Can you work these out from the drawing? Everything is in mm from the part's minimum corner. Coordinates: 2 decimals unless noted, no trailing zeros. Order: outer loops, then holes, each group sorted by start corner. A loop starts at its lowest first (then second) coordinate and runs counter-clockwise, first axis right, second up. Notation, with made-up numbers: M 11,11 L 25,11 A7 ccw 25,19 Z; hole C 85.5,20 d9. An arc over 180 degrees is marked long. Answer as CSV lines item,"result". Start each with the question number.
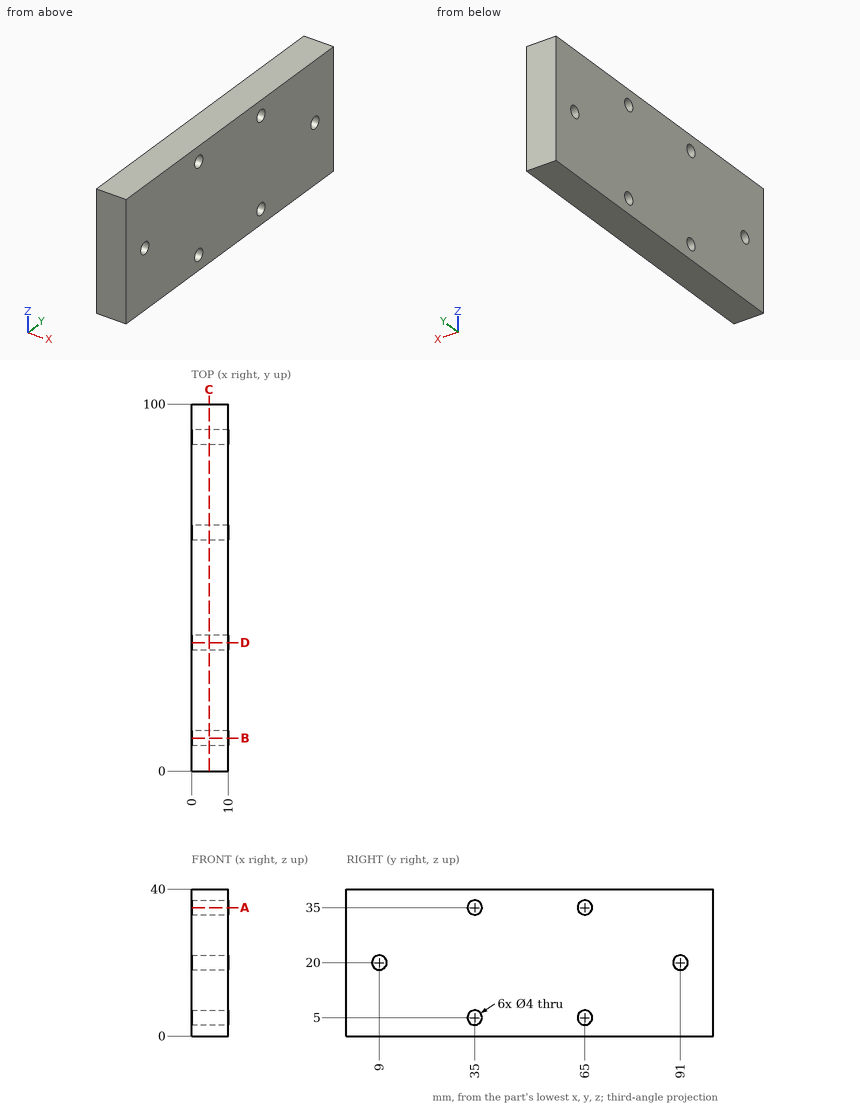
1) Suppose I cut it at B-B on y = 9. Please give me the cut outline in (x, z), plus the area to 3 significant figures.
2) Suppose I cut it at A-A on z = 35. Please give me the cut outline in (x, y).
3) Suppose I cut it at D-D on y = 35. Please give me the cut outline in (x, z), plus the area to 3 significant figures.
4) I need wall thicknesses on line 1 (Z direction, x = 4.5, y = 65); line 2 (Z direction, x = 7.25, y = 9); line 3 (Y direction, x = 1.5, z = 19.5). Which ranges of each line are inside material? Lowest first, please. Write a range as [from, to].
5) Suppose I cut it at C-C on x = 4.75. Please give me the cut outline in (y, z).
6) Will this pin go through, and if not, where does the flat tip stop? pin 1 Ø2.5 at (y, z) = (35, 5) entering from -X.
Output:
1,outline,"M 0,0 L 10,0 L 10,18 L 0,18 Z; M 0,22 L 10,22 L 10,40 L 0,40 Z"
1,area,"360 mm²"
2,outline,"M 0,0 L 10,0 L 10,33 L 0,33 Z; M 0,37 L 10,37 L 10,63 L 0,63 Z; M 0,67 L 10,67 L 10,100 L 0,100 Z"
3,outline,"M 0,0 L 10,0 L 10,3 L 0,3 Z; M 0,7 L 10,7 L 10,33 L 0,33 Z; M 0,37 L 10,37 L 10,40 L 0,40 Z"
3,area,"320 mm²"
4,line 1,"[0, 3], [7, 33], [37, 40]"
4,line 2,"[0, 18], [22, 40]"
4,line 3,"[0, 7.06], [10.94, 89.06], [92.94, 100]"
5,outline,"M 0,0 L 100,0 L 100,40 L 0,40 Z; hole C 9,20 d4; hole C 35,5 d4; hole C 35,35 d4; hole C 65,5 d4; hole C 65,35 d4; hole C 91,20 d4"
6,pin 1,"through"
